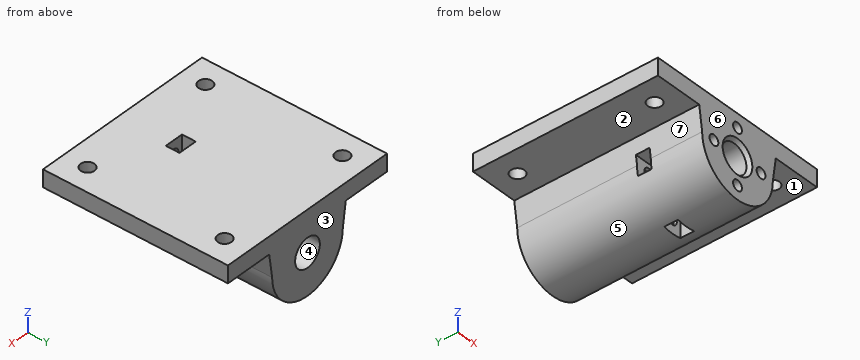
```python
from build123d import *

# Parameters (mm, degrees)
SZKIC1_R                    = 12
SZKIC1_R_2                  = 4.2
DODANIE_WYCI_GNI_CIE1_DEPTH = 54
DODANIE_WYCI_GNI_CIE2_DEPTH = 54
SZKIC4_R                    = 1.5
WYTNIJ_WYCI_GNI_CIE1_DEPTH  = 20
SZYK_KO_OWY1_COUNT          = 4
WYTNIJ_WYCI_GNI_CIE2_START  = -7
SZKIC5_W                    = 5.5
SZKIC5_H                    = 4
WYTNIJ_WYCI_GNI_CIE2_DEPTH  = 10
SZYK_KO_OWY2_COUNT          = 4
SFAZOWANIE1_SIZE            = 1
SFAZOWANIE1_SIZE2           = 0.839099631
WYTNIJ_WYCI_GNI_CIE3_REACH  = 66.969
SZKIC6_R                    = 2


with BuildPart() as part:
    # Szkic1 → Dodanie-wyciągnięcie1 (new body)
    with BuildSketch(Plane(origin=(0, 0, 0), x_dir=(1, 0, 0), z_dir=(0, 1, 0))):
        with Locations(Location((0, 12, 0), (0, 0, 270))):
            Circle(SZKIC1_R)
        with Locations(Location((0, 12, 0), (0, 0, 270))):
            Circle(SZKIC1_R_2, mode=Mode.SUBTRACT)
    extrude(amount=DODANIE_WYCI_GNI_CIE1_DEPTH)

    # Szkic3 → Dodanie-wyciągnięcie2 (add)
    with BuildSketch(Plane(origin=(0, 0, 0), x_dir=(1, 0, 0), z_dir=(0, 1, 0))):
        Polygon((0, 0), (27, 0), (27, 5), (13, 5), (12, 12), (0, 5.166487606), (-12, 12), (-13, 5), (-27, 5), (-27, 0), align=None)
    extrude(amount=DODANIE_WYCI_GNI_CIE2_DEPTH)

    # Szkic4 → Wytnij-wyciągnięcie1 (cut)
    with BuildSketch(Plane(origin=(0, 0, 0), x_dir=(-1, 0, 0), z_dir=(0, -1, 0))):
        with Locations(Location((0, 20, 0), (0, 0, 90))):
            Circle(SZKIC4_R)
    wytnij_wyci_gni_cie1 = extrude(amount=-WYTNIJ_WYCI_GNI_CIE1_DEPTH, mode=Mode.SUBTRACT)

    # Szyk kołowy1: Wytnij-wyciągnięcie1 ×4 about axis
    szyk_ko_owy1_axis = Axis((0, 0, -12), (0, 1, 0))
    for i in range(1, SZYK_KO_OWY1_COUNT):
        add(wytnij_wyci_gni_cie1.rotate(szyk_ko_owy1_axis, i * 360 / SZYK_KO_OWY1_COUNT), mode=Mode.SUBTRACT)

    # Szkic5 → Wytnij-wyciągnięcie2 (cut)
    with BuildSketch(Plane.XY.offset(WYTNIJ_WYCI_GNI_CIE2_START)):
        with Locations((0, 17)):
            Rectangle(SZKIC5_W, SZKIC5_H)
    wytnij_wyci_gni_cie2 = extrude(amount=WYTNIJ_WYCI_GNI_CIE2_DEPTH, mode=Mode.SUBTRACT)

    # Szyk kołowy2: Wytnij-wyciągnięcie2 ×4 about axis
    szyk_ko_owy2_axis = Axis((0, 0, -12), (0, 1, 0))
    for i in range(1, SZYK_KO_OWY2_COUNT):
        add(wytnij_wyci_gni_cie2.rotate(szyk_ko_owy2_axis, i * 360 / SZYK_KO_OWY2_COUNT), mode=Mode.SUBTRACT)

    # Sfazowanie1
    sfazowanie1_edges = [part.edges().sort_by_distance(p)[0] for p in [
        (0, 0, -16.2),
    ]]
    sfazowanie1_side = [part.faces().sort_by_distance(p)[0] for p in [
        (0, 27, -16.2),
    ]]
    chamfer(sfazowanie1_edges, length=SFAZOWANIE1_SIZE, length2=SFAZOWANIE1_SIZE2, reference=sfazowanie1_side[0])

    # Szkic6 → Wytnij-wyciągnięcie3 (cut, up to next)
    with BuildSketch(Plane.XY, mode=Mode.PRIVATE) as wytnij_wyci_gni_cie3_sk1:
        with Locations((-20, 47)):
            Circle(SZKIC6_R)
    wytnij_wyci_gni_cie3_tool1 = extrude(wytnij_wyci_gni_cie3_sk1.sketch, amount=-WYTNIJ_WYCI_GNI_CIE3_REACH, mode=Mode.PRIVATE) & part.part
    # Szkic6 → Wytnij-wyciągnięcie3 (cut, up to next)
    with BuildSketch(Plane.XY, mode=Mode.PRIVATE) as wytnij_wyci_gni_cie3_sk2:
        with Locations((20, 47)):
            Circle(SZKIC6_R)
    wytnij_wyci_gni_cie3_tool2 = extrude(wytnij_wyci_gni_cie3_sk2.sketch, amount=-WYTNIJ_WYCI_GNI_CIE3_REACH, mode=Mode.PRIVATE) & part.part
    # Szkic6 → Wytnij-wyciągnięcie3 (cut, up to next)
    with BuildSketch(Plane.XY, mode=Mode.PRIVATE) as wytnij_wyci_gni_cie3_sk3:
        with Locations((20, 7)):
            Circle(SZKIC6_R)
    wytnij_wyci_gni_cie3_tool3 = extrude(wytnij_wyci_gni_cie3_sk3.sketch, amount=-WYTNIJ_WYCI_GNI_CIE3_REACH, mode=Mode.PRIVATE) & part.part
    # Szkic6 → Wytnij-wyciągnięcie3 (cut, up to next)
    with BuildSketch(Plane.XY, mode=Mode.PRIVATE) as wytnij_wyci_gni_cie3_sk4:
        with Locations((-20, 7)):
            Circle(SZKIC6_R)
    wytnij_wyci_gni_cie3_tool4 = extrude(wytnij_wyci_gni_cie3_sk4.sketch, amount=-WYTNIJ_WYCI_GNI_CIE3_REACH, mode=Mode.PRIVATE) & part.part
    add(wytnij_wyci_gni_cie3_tool1.solids().sort_by_distance((-20, 47, 0))[0], mode=Mode.SUBTRACT)
    add(wytnij_wyci_gni_cie3_tool2.solids().sort_by_distance((20, 47, 0))[0], mode=Mode.SUBTRACT)
    add(wytnij_wyci_gni_cie3_tool3.solids().sort_by_distance((20, 7, 0))[0], mode=Mode.SUBTRACT)
    add(wytnij_wyci_gni_cie3_tool4.solids().sort_by_distance((-20, 7, 0))[0], mode=Mode.SUBTRACT)


solid = part.part
```
The listing builds one solid part. Answer for the finished solid, in the listing's coordinates (mm). Face numbers are marked on the shaded views. A direction names the side the tool comes from. Round coordinates to 2 decimals unless told otherwise and drop trailing zeros. Write each loop counter-clockwise with the first axis right and the second up, starting at its lowest first coordinate (ties: lowest second). Pieces come first, ordered by that corner, then holes. Notation, with made-up numbers: (83.5, 42) -> (87.5, 42) arc R18 cw to (87.5, 56) -> close; hole circle Ø5 at (-2.75, -28). An arc over 180 degrees is marked (long way). Use CSV: the item, a comma, the result in double quotes. Start each with the question number.
(1) Each of these flat-tipped pins is pushed along its axis until it touches: pin 1 (3 mm diameter, centred on y = 20.5, z = -12, fed in from -X); pin 2 (4 mm diameter, centred on x = 23, y = 29, fed in from -Z); pin 3 (2.5 mm diameter, centred on x = 0, z = -4, fed in from -Y). Where does it stop, or does it pass through?
(2) The mould has two halves that part along X. Classify the marked faces 4, 5, 6 and 7: released by +X, released by -X, zero draft, split by the parting line, or undercut.
(3) Section C-C on y = 16 is taken. Give the vertices of the cut face in (x, z).
(4) Section B-B on x = 0 is taken. Count the separate pieces of the cut face and the enclosed holes in it, then the cut area to 3 significant figures.
(5) Section A-A on y = 7 is taken. Give the vertices of the cut face in (x, z).
(6) Section D-D on z = -17.75 is taken. Give the vertices of the cut face in (x, y).
(7) Which of the six approach directions +Z, -Z, +X, -X, +Y, -Y give full straight-line access (tool end or side, diameter ignored) to the marked faces 1, 2 and 3?
(8) Consider L1, parallel to Y at x = 20, z = -2.65; L2, parallel to Y at x = -0.5, z = -2.5; L3, parallel to X at y = 34, z = -8.25. Determine where each line is inside the solid, lowest interval first. Write a range as from..to.
A:
1,pin 1,"stops at x = -12.21"
1,pin 2,"stops at z = -5"
1,pin 3,"stops at y = 20"
2,face 4,"undercut"
2,face 5,"split by the parting line"
2,face 6,"zero draft"
2,face 7,"released by -X"
3,outline,"(-27, -5) -> (-13, -5) -> (-12.39, -9.25) -> (-5, -9.25) -> (-5, -14.75) -> (-11.68, -14.75) arc R12 ccw to (-2.75, -23.68) -> (-2.75, -17) -> (2.75, -17) -> (2.75, -23.68) arc R12 ccw to (11.68, -14.75) -> (5, -14.75) -> (5, -9.25) -> (12.39, -9.25) -> (13, -5) -> (27, -5) -> (27, 0) -> (2.75, 0) -> (2.75, -7) -> (-2.75, -7) -> (-2.75, 0) -> (-27, 0) -> close; hole circle Ø8.4 at (0, -12)"
4,separate pieces,"4"
4,enclosed holes,"0"
4,area,"690 mm²"
5,outline,"(-27, -5) -> (-22, -5) -> (-22, 0) -> (-27, 0) -> close; (-18, -5) -> (-13, -5) -> (-12, -12) arc R12 ccw to (12, -12) -> (13, -5) -> (18, -5) -> (18, 0) -> (-18, 0) -> close; (22, -5) -> (27, -5) -> (27, 0) -> (22, 0) -> close; hole circle Ø3 at (-8, -12); hole circle Ø8.4 at (0, -12); hole circle Ø3 at (0, -20); hole circle Ø3 at (0, -4); hole circle Ø3 at (8, -12)"
6,outline,"(-10.53, 0) -> (10.53, 0) -> (10.53, 54) -> (-10.53, 54) -> close; hole (-2.75, 15) -> (2.75, 15) -> (2.75, 19) -> (-2.75, 19) -> close"
7,face 1,"-Z, +X, +Y, -Y"
7,face 2,"-Z, -X, +Y, -Y"
7,face 3,"+Z, -Z, +X, -X, +Y"
8,L1,"y = 0..5, 9..45, 49..54"
8,L2,"y = 0..15, 19..54"
8,L3,"x = -12.54..-1.89, 1.89..12.54"
